For this review, take the finished solid that the model builds, in its own axes (mm). A direction names the side the tool comes from. Round coordinates to 2 decimals unless told otherwise and drop trailing zeros. Loops run counter-clockwise (first coordinate to the right, second up) from the corner with the lowest first, then second, coordinate; pieces in that order, holes last.
```python
from build123d import *

# Parameters (mm, degrees)
F0_DEPTH       = 70
F1_W           = 65
F1_H           = 16.5
F8_DEPTH       = 2
F2_T1_DEPTH    = 12.5
F2_T3_DEPTH    = 73
F2_T5_DEPTH    = 57
F2_T7_DEPTH    = 61
F2_S11_W       = 2.04
F2_S11_H       = 2.04
F2_T12_DEPTH   = 2.04
F2_S17_W       = 2.04
F2_S17_H       = 2.04
F2_T18_DEPTH   = 2.04
F2_S23_W       = 2.04
F2_S23_H       = 2.04
F2_T24_DEPTH   = 2.04
F2_S29_W       = 2.04
F2_S29_H       = 2.04
F2_T30_DEPTH   = 2.04
F2_T37_DEPTH   = 73
F2_T42_DEPTH   = 62
F2_T50_DEPTH   = 62
F2_T55_DEPTH   = 73
F2_T62_DEPTH   = 17.5
F2_T67_DEPTH   = 17.5
F5_D           = 3.2
F5_CSINK_D     = 5.5
F5_CSINK_ANGLE = 90
F6_D           = 3.2
F6_CSINK_D     = 5.5
F6_CSINK_ANGLE = 90


# Not quite as in the source:
# - a fillet or chamfer that OpenCascade refuses, or shapes differently, is made with other operations: its cross-section is extruded or revolved along the edge and cut away or added
# - a feature names something its author has since deleted; it is built from what else it names


with BuildPart() as f0:
    # F7 (on Top) → F0 (new body)
    with BuildSketch(Plane.XY):
        Polygon((-32.5, 16.5), (-32.5, 0), (32.5, 0), (32.5, 16.5), (28.5, 16.5), (28.5, 14.5), (30.5, 14.5), (30.5, 2), (-30.5, 2), (-30.5, 14.5), (-28.5, 14.5), (-28.5, 16.5), align=None)
    extrude(amount=F0_DEPTH)

    # F1 (on face) → F8 (join)
    with BuildSketch(Plane(origin=(0, 0, 0), x_dir=(1, 0, 0), z_dir=(0, 0, -1))):
        with Locations((0, -8.25)):
            Rectangle(F1_W, F1_H)
    extrude(amount=-F8_DEPTH)

    # F2: fillet of radius 2 on 13 edges, made by hand

    # F2_s2 → F2_t1 (cut)
    with BuildSketch(Plane.XZ.offset(-14.5)):
        with BuildLine():
            ThreePointArc((32.5, 2), (31.9142135624, 0.5857864376), (30.5, 0))
            Line((30.5, 0), (32.5, 0))
            Line((32.5, 0), (32.5, 2))
        make_face()
        with BuildLine():
            ThreePointArc((-32.5, 2), (-31.9142135624, 0.5857864376), (-30.5, 0))
            Line((-30.5, 0), (-32.5, 0))
            Line((-32.5, 0), (-32.5, 2))
        make_face()
    extrude(amount=F2_T1_DEPTH, mode=Mode.SUBTRACT)

    # F2_s4 → F2_t3 (cut)
    with BuildSketch(Plane.XY.offset(2)):
        with BuildLine():
            ThreePointArc((-32.5, 2), (-31.9142135624, 0.5857864376), (-30.5, 0))
            Line((-30.5, 0), (-32.5, 0))
            Line((-32.5, 0), (-32.5, 2))
        make_face()
        with BuildLine():
            ThreePointArc((30.5, 0), (31.9142135624, 0.5857864376), (32.5, 2))
            Line((32.5, 2), (32.5, 0))
            Line((32.5, 0), (30.5, 0))
        make_face()
        with BuildLine():
            ThreePointArc((-32.5, 14.5), (-31.9142135624, 15.9142135624), (-30.5, 16.5))
            Line((-30.5, 16.5), (-32.5, 16.5))
            Line((-32.5, 16.5), (-32.5, 14.5))
        make_face()
        with BuildLine():
            ThreePointArc((32.5, 14.5), (31.9142135624, 15.9142135624), (30.5, 16.5))
            Line((30.5, 16.5), (32.5, 16.5))
            Line((32.5, 16.5), (32.5, 14.5))
        make_face()
        with BuildLine():
            ThreePointArc((-28.5, 14.5), (-29.0857864376, 15.9142135624), (-30.5, 16.5))
            Line((-30.5, 16.5), (-28.5, 16.5))
            Line((-28.5, 16.5), (-28.5, 14.5))
        make_face()
        with BuildLine():
            ThreePointArc((28.5, 14.5), (29.0857864376, 15.9142135624), (30.5, 16.5))
            Line((30.5, 16.5), (28.5, 16.5))
            Line((28.5, 16.5), (28.5, 14.5))
        make_face()
    extrude(amount=F2_T3_DEPTH, mode=Mode.SUBTRACT)

    # F2_s6 → F2_t5 (cut)
    with BuildSketch(Plane.YZ.offset(-28.5)):
        with BuildLine():
            ThreePointArc((14.5, 2), (15.9142135624, 1.4142135624), (16.5, 0))
            Line((16.5, 0), (16.5, 2))
            Line((16.5, 2), (14.5, 2))
        make_face()
    extrude(amount=F2_T5_DEPTH, mode=Mode.SUBTRACT)

    # F2_s8 → F2_t7 (cut)
    with BuildSketch(Plane.YZ.offset(-30.5)):
        with BuildLine():
            ThreePointArc((0, 2), (0.5857864376, 0.5857864376), (2, 0))
            Line((2, 0), (0, 0))
            Line((0, 0), (0, 2))
        make_face()
        with BuildLine():
            ThreePointArc((16.5, 2), (15.9142135624, 0.5857864376), (14.5, 0))
            Line((14.5, 0), (16.5, 0))
            Line((16.5, 0), (16.5, 2))
        make_face()
    extrude(amount=F2_T7_DEPTH, mode=Mode.SUBTRACT)


with BuildPart() as f2_tool10:
    # F2_s11 → F2_t12 (new body)
    with BuildSketch(Plane.XZ.offset(-2)):
        with Locations((31.52, 0.98)):
            Rectangle(F2_S11_W, F2_S11_H)
    extrude(amount=F2_T12_DEPTH)

    # F2_s13 → F2_t14 (revolve, cut)
    with BuildSketch(Plane(origin=(30.5, 2, 2), x_dir=(-0.7071067812, 0, 0.7071067812), z_dir=(0.7071067812, 0, 0.7071067812))):
        with BuildLine():
            ThreePointArc((0, -2), (2, 0), (0, 2))
            Line((0, 2), (0, -2))
        make_face()
    revolve(axis=Axis((30.5, 2, 2), (0, -1, 0)), mode=Mode.SUBTRACT)


with BuildPart() as f0_1:
    add(f0.part)

    # F2_t9: cut F2_tool10
    add(f2_tool10.part, mode=Mode.SUBTRACT)


with BuildPart() as f2_tool16:
    # F2_s17 → F2_t18 (new body)
    with BuildSketch(Plane.YZ.offset(30.5)):
        with Locations((15.52, 0.98)):
            Rectangle(F2_S17_W, F2_S17_H)
    extrude(amount=F2_T18_DEPTH)

    # F2_s19 → F2_t20 (revolve, cut)
    with BuildSketch(Plane(origin=(30.5, 14.5, 2), x_dir=(0, -0.7071067812, 0.7071067812), z_dir=(0, 0.7071067812, 0.7071067812))):
        with BuildLine():
            ThreePointArc((0, -2), (2, 0), (0, 2))
            Line((0, 2), (0, -2))
        make_face()
    revolve(axis=Axis((30.5, 14.5, 2), (1, 0, 0)), mode=Mode.SUBTRACT)


with BuildPart() as f0_2:
    add(f0_1.part)

    # F2_t15: cut F2_tool16
    add(f2_tool16.part, mode=Mode.SUBTRACT)


with BuildPart() as f2_tool22:
    # F2_s23 → F2_t24 (new body)
    with BuildSketch(Plane.YZ.offset(-30.5)):
        with Locations((15.52, 0.98)):
            Rectangle(F2_S23_W, F2_S23_H)
    extrude(amount=-F2_T24_DEPTH)

    # F2_s25 → F2_t26 (revolve, cut)
    with BuildSketch(Plane(origin=(-30.5, 14.5, 2), x_dir=(0, -0.7071067812, 0.7071067812), z_dir=(0, -0.7071067812, -0.7071067812))):
        with BuildLine():
            ThreePointArc((0, -2), (2, 0), (0, 2))
            Line((0, 2), (0, -2))
        make_face()
    revolve(axis=Axis((-30.5, 14.5, 2), (-1, 0, 0)), mode=Mode.SUBTRACT)


with BuildPart() as f0_3:
    add(f0_2.part)

    # F2_t21: cut F2_tool22
    add(f2_tool22.part, mode=Mode.SUBTRACT)


with BuildPart() as f2_tool28:
    # F2_s29 → F2_t30 (new body)
    with BuildSketch(Plane.YZ.offset(-30.5)):
        with Locations((0.98, 0.98)):
            Rectangle(F2_S29_W, F2_S29_H)
    extrude(amount=-F2_T30_DEPTH)

    # F2_s31 → F2_t32 (revolve, cut)
    with BuildSketch(Plane(origin=(-30.5, 2, 2), x_dir=(0, 0.7071067812, 0.7071067812), z_dir=(0, -0.7071067812, 0.7071067812))):
        with BuildLine():
            ThreePointArc((0, -2), (2, 0), (0, 2))
            Line((0, 2), (0, -2))
        make_face()
    revolve(axis=Axis((-30.5, 2, 2), (-1, 0, 0)), mode=Mode.SUBTRACT)


with BuildPart() as f0_4:
    add(f0_3.part)

    # F2_t27: cut F2_tool28
    add(f2_tool28.part, mode=Mode.SUBTRACT)


with BuildPart() as f2_tool35:
    # F2_s36 → F2_t37 (new body)
    with BuildSketch(Plane.XY.offset(-3)):
        with BuildLine():
            ThreePointArc((-28.5, 14.5), (-29.0857864376, 15.9142135624), (-30.5, 16.5))
            Line((-30.5, 16.5), (-28.5, 16.5))
            Line((-28.5, 16.5), (-28.5, 14.5))
        make_face()
    extrude(amount=F2_T37_DEPTH)

    split(bisect_by=Plane.XY.offset(2), keep=Keep.BOTTOM)

    split(bisect_by=Plane.XY, keep=Keep.TOP)


with BuildPart() as f2_tool40:
    # F2_s41 → F2_t42 (new body)
    with BuildSketch(Plane.YZ.offset(-33.5)):
        with BuildLine():
            ThreePointArc((14.5, 2), (15.9142135624, 1.4142135624), (16.5, 0))
            Line((16.5, 0), (16.5, 2))
            Line((16.5, 2), (14.5, 2))
        make_face()
    extrude(amount=F2_T42_DEPTH)

    split(bisect_by=Plane.YZ.offset(-28.5), keep=Keep.BOTTOM)

    split(bisect_by=Plane.YZ.offset(-30.5), keep=Keep.TOP)


with BuildPart() as f2_tool35_1:
    add(f2_tool35.part)

    # F2_t45: intersect F2_tool40
    add(f2_tool40.part, mode=Mode.INTERSECT)


with BuildPart() as f0_5:
    add(f0_4.part)

    # F2_t33: cut F2_tool35
    add(f2_tool35_1.part, mode=Mode.SUBTRACT)


with BuildPart() as f2_tool48:
    # F2_s49 → F2_t50 (new body)
    with BuildSketch(Plane.YZ.offset(-28.5)):
        with BuildLine():
            ThreePointArc((14.5, 2), (15.9142135624, 1.4142135624), (16.5, 0))
            Line((16.5, 0), (16.5, 2))
            Line((16.5, 2), (14.5, 2))
        make_face()
    extrude(amount=F2_T50_DEPTH)

    split(bisect_by=Plane.YZ.offset(30.5), keep=Keep.BOTTOM)

    split(bisect_by=Plane.YZ.offset(28.5), keep=Keep.TOP)


with BuildPart() as f2_tool53:
    # F2_s54 → F2_t55 (new body)
    with BuildSketch(Plane.XY.offset(-3)):
        with BuildLine():
            ThreePointArc((28.5, 14.5), (29.0857864376, 15.9142135624), (30.5, 16.5))
            Line((30.5, 16.5), (28.5, 16.5))
            Line((28.5, 16.5), (28.5, 14.5))
        make_face()
    extrude(amount=F2_T55_DEPTH)

    split(bisect_by=Plane.XY.offset(2), keep=Keep.BOTTOM)

    split(bisect_by=Plane.XY, keep=Keep.TOP)


with BuildPart() as f2_tool48_1:
    add(f2_tool48.part)

    # F2_t58: intersect F2_tool53
    add(f2_tool53.part, mode=Mode.INTERSECT)


with BuildPart() as f0_6:
    add(f0_5.part)

    # F2_t46: cut F2_tool48
    add(f2_tool48_1.part, mode=Mode.SUBTRACT)


with BuildPart() as f2_tool60:
    # F2_s61 → F2_t62 (new body)
    with BuildSketch(Plane.XZ.offset(3)):
        with BuildLine():
            ThreePointArc((30.5, 4), (29.9142135624, 2.5857864376), (28.5, 2))
            Line((28.5, 2), (30.5, 2))
            Line((30.5, 2), (30.5, 4))
        make_face()
    extrude(amount=-F2_T62_DEPTH)

    split(bisect_by=Plane.XZ, keep=Keep.BOTTOM)


with BuildPart() as f0_7:
    add(f0_6.part)

    # F2_t59: union F2_tool60
    add(f2_tool60.part)


with BuildPart() as f2_tool65:
    # F2_s66 → F2_t67 (new body)
    with BuildSketch(Plane.XZ.offset(-14.5)):
        with BuildLine():
            ThreePointArc((-30.5, 4), (-29.9142135624, 2.5857864376), (-28.5, 2))
            Line((-28.5, 2), (-30.5, 2))
            Line((-30.5, 2), (-30.5, 4))
        make_face()
    extrude(amount=F2_T67_DEPTH)

    split(bisect_by=Plane.XZ, keep=Keep.BOTTOM)


with BuildPart() as f0_8:
    add(f0_7.part)

    # F2_t64: union F2_tool65
    add(f2_tool65.part)

    # F5 (through all)
    with Locations(Plane(origin=(0, 2, 0), x_dir=(-1, 0, 0), z_dir=(0, 1, 0))):
        with Locations((0, 18)):
            CounterSinkHole(F5_D / 2, F5_CSINK_D / 2, counter_sink_angle=F5_CSINK_ANGLE)

    # F6 (through all)
    with Locations(Plane(origin=(0, 2, 0), x_dir=(-1, 0, 0), z_dir=(0, 1, 0))):
        with Locations((0, 10)):
            CounterSinkHole(F6_D / 2, F6_CSINK_D / 2, counter_sink_angle=F6_CSINK_ANGLE)


solid = f0_8.part
```
(1) For L1, parallel to X at y = 14, z = 55; L2, parallel to Z at x = 0, y = 0.6; L3, parallel to Z at x = 0, y = 0.65, list the stretches that pass through material, from the lowest coordinate up.
(2) For faces 1 (the cylindrical face through (31.9, 0.57, 35.52)), 2 (the cylindrical face through (-29.93, 8.34, 2.6)), 3 (the cylindrical face through (-0.41, 15.49, 1.74)), list the 3-axis set-ups (+Z, -Z, +X, -X, +Y, -Y) from which the entire face can be reached by the end or side of a thin tool; tool diameter is ignored.
(3) Add section C-C (y = 5). Give the boundary of the cut face in (x, z), plus the area to 3 significant figures.
(4) Add section B-B (x = 0). Give the boundary of the cut face in (y, z).
(5) Add section D-D (x = 18.5). Give the boundary of the cut face in (y, z), plus the area to 3 significant figures.
(6) Add section A-A (z = 10). Give the boundary of the cut face in (x, y), plus the area to 3 significant figures.
(7) Insertion check: pin 1 Ø5 at (x, y) = (18.5, 7.5) entering from +Z; pin 2 Ø10 at (x, z) = (-19, 51.5) entering from +Y; pin 3 Ø4 at (x, z) = (0, 10) entering from +Y; pin 4 Ø1.9 at (x, z) = (0, 18) entering from +Y. Each pin has a flat end and moves straight along its axis. Give the tip position at first contact, or say it passes through.
(8) The part is to be moulded in two halves that separate along Z. For faces 4 (the cylindrical face through (-0.35, 0.42, 8.44)), 5 (the cylindrical face through (-0.208, 0.419, 19.586)), 6 (the flat face through (0, 8, 0)), 7 (the flat face through (0, 0, 36)), say which applies: pulls with the +Z half, pulls with the -Z half, needs draft (parallel to the pull), parting line crosses it, or undercut.
Outcome:
1. L1: x = -32.5 to -30.5, 30.5 to 32.5
1. L2: z = 0.57 to 8.4, 11.6 to 16.4, 19.6 to 70
1. L3: z = 0.52 to 8.4, 11.6 to 16.4, 19.6 to 70
2. face 1: +Z, -Z, +X, -Y
2. face 2: +Z
2. face 3: +Z, +Y
3. outline: (-32.5, 2) arc R2 ccw to (-30.5, 0) - (30.5, 0) arc R2 ccw to (32.5, 2) - (32.5, 70) - (30.5, 70) - (30.5, 4) arc R2 cw to (28.5, 2) - (-28.5, 2) arc R2 cw to (-30.5, 4) - (-30.5, 70) - (-32.5, 70) - close
3. area: 402 mm2
4. outline: (0, 2) arc R2 ccw to (2, 0) - (14.5, 0) arc R2 ccw to (16.23, 1) arc R2 ccw to (14.5, 2) - (2, 2) - (2, 7.25) - (0.85, 8.4) - (0, 8.4) - close; (0, 11.6) - (0.85, 11.6) - (2, 12.75) - (2, 15.25) - (0.85, 16.4) - (0, 16.4) - close; (0, 19.6) - (0.85, 19.6) - (2, 20.75) - (2, 70) - (0, 70) - close
5. outline: (0, 2) arc R2 ccw to (2, 0) - (14.5, 0) arc R2 ccw to (16.23, 1) arc R2 ccw to (14.5, 2) - (2, 2) - (2, 70) - (0, 70) - close
5. area: 167 mm2
6. outline: (-32.5, 2) arc R2 ccw to (-30.5, 0) - (-1.6, 0) - (-1.6, 0.85) - (-2.75, 2) - (-30.5, 2) - (-30.5, 14.5) - (-28.5, 14.5) arc R2 ccw to (-32.5, 14.5) - close; (1.6, 0) - (30.5, 0) arc R2 ccw to (32.5, 2) - (32.5, 14.5) arc R2 ccw to (28.5, 14.5) - (30.5, 14.5) - (30.5, 2) - (2.75, 2) - (1.6, 0.85) - close
6. area: 183 mm2
7. pin 1: stops at z = 2
7. pin 2: stops at y = 2
7. pin 3: stops at y = 1.25
7. pin 4: passes through
8. face 4: undercut
8. face 5: undercut
8. face 6: pulls with the -Z half
8. face 7: needs draft
